Source: CAD feature listing. Evaluate the final solid. Frame: model axes, mm. Face numbers are marked on the shaded views. A direction names the side the tool comes from. Give positions to 0.01 mm unless a question says otherwise; leave off trailing zeros. Order: outer loops, then holes, each group sorted by start corner. A loop starts at its lowest first (then second) coordinate and runs counter-clockwise, first axis right, second up. Notation, with made-up numbers: (-36, 19) -> (21, 19) arc R33 ccw to (21, 47) -> close; hole circle Ø3 at (3, 48). An arc over 180 degrees is marked (long way). Answer in a Markdown table with one row per item.
```python
from build123d import *

# Parameters (mm, degrees)
BOSS_EXTRUDE1_DEPTH             = 10
TAP_DRILL_FOR_M4X0_7_TAP1_D     = 3.3
TAP_DRILL_FOR_M4X0_7_TAP1_DEPTH = 9.7
SKETCH5_W                       = 2.4
SKETCH5_H                       = 9.7
TAP_DRILL_FOR_M4X0_7_TAP2_D     = 3.3
FILLET1_R                       = 1


with BuildPart() as part:
    # Sketch1 → Boss-Extrude1 (new body)
    with BuildSketch(Plane(origin=(0, 0, 0), x_dir=(1, 0, 0), z_dir=(0, 1, 0))):
        Polygon((-3.3, 3.3), (-3.3, -13.3), (-13, -13.3), (-13, 13), (13, 13), (13, -13.3), (3.3, -13.3), (3.3, 3.3), align=None)
    extrude(amount=BOSS_EXTRUDE1_DEPTH)

    # Tap Drill for M4x0.7 Tap1
    with Locations(Plane(origin=(-13, 5, 8.3), x_dir=(0, 0, -1), z_dir=(-1, 0, 0))):
        with Locations((0, 0)):
            Hole(TAP_DRILL_FOR_M4X0_7_TAP1_D / 2, depth=TAP_DRILL_FOR_M4X0_7_TAP1_DEPTH)

    # Sketch5 → M4 Clearance Hole1 (revolve, cut)
    with BuildSketch(Plane(origin=(3.3, 5, 8.3), x_dir=(0, 0, 1), z_dir=(0, 1, 0))):
        with Locations((1.2, 4.85)):
            Rectangle(SKETCH5_W, SKETCH5_H)
    revolve(axis=Axis((-3.05, 5, 8.3), (1, 0, 0)), mode=Mode.SUBTRACT)

    # Tap Drill for M4x0.7 Tap2 (through all)
    with Locations(Plane(origin=(0, 5, -13), x_dir=(-1, 0, 0), z_dir=(0, 0, -1))):
        with Locations((0, 0)):
            Hole(TAP_DRILL_FOR_M4X0_7_TAP2_D / 2)

    # Fillet1
    fillet1_edges = [part.edges().sort_by_distance(p)[0] for p in [
        (-13, 5, -13),
        (13, 5, -13),
    ]]
    fillet(fillet1_edges, radius=FILLET1_R)


solid = part.part
```
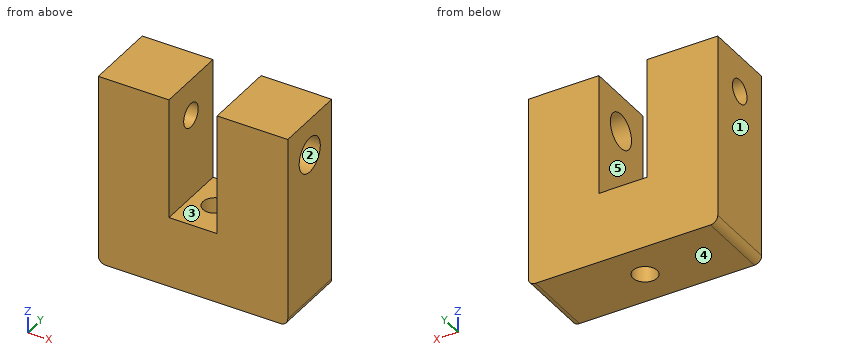
(1) Ray query, probe 1 along X at (y, z) = (2.75, 9.75); probe 2 along Z at (x, y) = (7.25, 5); probe 3 along Z at (x, y) = (-11, 5). Return the intervals inside material, ascending.
A:
| item | result |
|---|---|
| probe 1 | x = -13 to -3.3, 3.3 to 13 |
| probe 2 | z = -13 to 5.9, 10.7 to 13.3 |
| probe 3 | z = -13 to 6.65, 9.95 to 13.3 |
(2) Section query C-C (y = 4). Return the cut outline in (x, z).
A:
| item | result |
|---|---|
| outline | (-13, -12) arc R1 ccw to (-12, -13) -> (-1.31, -13) -> (-1.31, -3.3) -> (-3.3, -3.3) -> (-3.3, 6.99) -> (-13, 6.99) -> close; (-13, 9.61) -> (-3.3, 9.61) -> (-3.3, 13.3) -> (-13, 13.3) -> close; (1.31, -13) -> (12, -13) arc R1 ccw to (13, -12) -> (13, 6.12) -> (3.3, 6.12) -> (3.3, -3.3) -> (1.31, -3.3) -> close; (3.3, 10.48) -> (13, 10.48) -> (13, 13.3) -> (3.3, 13.3) -> close |
(3) Pull-direction query (X, two-part tool) for the marked faces 1, 2 and 3; classes: +X half, -X half, draft (parallel to the pull), parting line (faces both ways), or undercut.
A:
| item | result |
|---|---|
| face 1 | -X half |
| face 2 | draft |
| face 3 | undercut |
(4) Access query for the marked faces 4 and 5. Directions: +Z, -Z, +X, -X, +Y, -Y. A direction counts if a zero-diameter tool reaches every point of the face in a straight line with its end or side. Return the directions, or none.
A:
| item | result |
|---|---|
| face 4 | -Z, +X, -X, +Y, -Y |
| face 5 | +Z, +Y, -Y |
(5) Section query D-D (y = 7). Return the cut outline in (x, z).
A:
| item | result |
|---|---|
| outline | (-13, -12) arc R1 ccw to (-12, -13) -> (12, -13) arc R1 ccw to (13, -12) -> (13, 6.97) -> (3.3, 6.97) -> (3.3, -3.3) -> (-3.3, -3.3) -> (-3.3, 13.3) -> (-13, 13.3) -> close; (3.3, 9.63) -> (13, 9.63) -> (13, 13.3) -> (3.3, 13.3) -> close |
(6) First-contact query: pin 1 Ø3 at (y, z) = (5, 8.3) entering from +X; pin 2 Ø3.5 at (x, y) = (0.5, 6) entering from +Z. Flat tips, straight axial feed; report the tip coordinate or a pass-through.
A:
| item | result |
|---|---|
| pin 1 | passes through |
| pin 2 | stops at z = -3.3 |
(7) Section query B-B (z = 8.3). Return the cut outline in (x, y), plus the area to 3 significant figures.
A:
| item | result |
|---|---|
| outline | (-13, 0) -> (-3.3, 0) -> (-3.3, 3.35) -> (-13, 3.35) -> close; (-13, 6.65) -> (-3.3, 6.65) -> (-3.3, 10) -> (-13, 10) -> close; (3.3, 0) -> (13, 0) -> (13, 2.6) -> (3.3, 2.6) -> close; (3.3, 7.4) -> (13, 7.4) -> (13, 10) -> (3.3, 10) -> close |
| area | 115 mm^2 |
(8) Section query A-A (x = 0). Return the cut outline in (y, z).
A:
| item | result |
|---|---|
| outline | (0, -13) -> (3.35, -13) -> (3.35, -3.3) -> (0, -3.3) -> close; (6.65, -13) -> (10, -13) -> (10, -3.3) -> (6.65, -3.3) -> close |
